from build123d import *

# Parameters (mm, degrees)
F0_R     = 50
F1_DEPTH = 10
F2_R     = 50
F2_R_2   = 45
F3_DEPTH = 200
F4_R     = 2.5
F5_DEPTH = 20


with BuildPart() as f1:
    # F0 (on Top) → F1 (new body)
    with BuildSketch(Plane.XY):
        Circle(F0_R)
    extrude(amount=F1_DEPTH)

    # F2 (on face) → F3 (join)
    with BuildSketch(Plane(origin=(0, 0, 0), x_dir=(1, 0, 0), z_dir=(0, 0, -1))):
        Circle(F2_R)
        Circle(F2_R_2, mode=Mode.SUBTRACT)
    extrude(amount=F3_DEPTH)

    # F4 (on face) → F5 (join)
    with BuildSketch(Plane.XY.offset(10)):
        Circle(F4_R)
        with Locations((-10, 0)):
            Circle(F4_R)
        with Locations((0, 10)):
            Circle(F4_R)
        with Locations((10, 0)):
            Circle(F4_R)
        with Locations((0, -10)):
            Circle(F4_R)
    extrude(amount=F5_DEPTH)


solid = f1.part
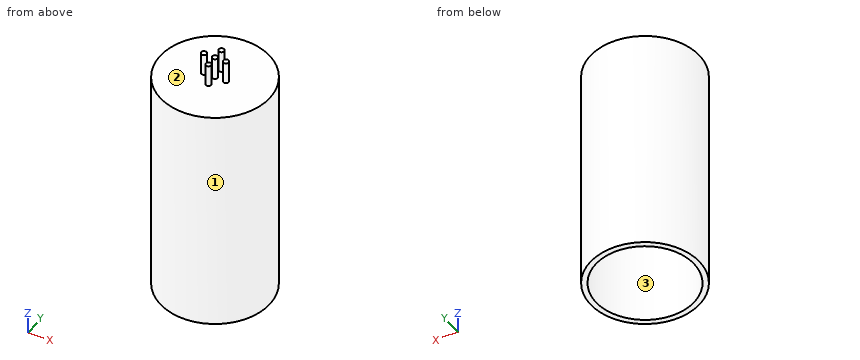
Input: part model. Units: mm. Frame: model coordinates. Face numbers are marked on the shaded views. A direction names the side the tool comes from. Coordinates: 2 decimals unless noted, no trailing zeros. Loops run counter-clockwise (first coordinate to the right, second up) from the corner with the lowest first, then second, coordinate; pieces in that order, holes last.
Q1. Material intervals for line 1 (Y direction, x = 0, z = -72); line 2 (Z direction, x = 2.5, y = -26.5), sorted ascending.
Q2. Cut plane D-D (z = 3). Output: boundary loops of the cut face in (x, y).
Q3. Cut plane B-B (y = 10). Output: boundary loops of the cut face in (x, z), then the cut area to 3 significant figures.
Q4. Set-up query: the marked faces 1, 2 and 3. Return all of +Z, -Z, +X, -X, +Y, -Y with unobstructed straight access to the full face (end or side cutting, diameter ignored); none if empty.
Q5. Cut plane A-A (x = 0). Output: boundary loops of the cut face in (y, z), then the cut area to 3 significant figures.
Q6. Cut plane C-C (z = -149.5). Output: boundary loops of the cut face in (x, y), then the cut area to 3 significant figures.
Q7. Contact query for flat-ended pins moving along their axis: pin 1 (12 mm diameter, centred on x = -29, z = -82, fed in from -Y); pin 2 (1 mm diameter, centred on x = 3, z = -148, fed in from +Y); pin 3 (4 mm diameter, centred on x = 15, y = -21, fed in from -Z). Output: stop coordinate, or through.
Working result:
1. line 1: y = -50 to -45, 45 to 50
1. line 2: z = 0 to 10
2. outline: circle Ø100 at (0, 0)
3. outline: (-48.99, -200) - (-43.87, -200) - (-43.87, 0) - (43.87, 0) - (43.87, -200) - (48.99, -200) - (48.99, 10) - (2.5, 10) - (2.5, 30) - (-2.5, 30) - (-2.5, 10) - (-48.99, 10) - close
3. area: 3,130 mm2
4. face 1: +Z, -Z
4. face 2: +Z
4. face 3: -Z
5. outline: (-50, -200) - (-45, -200) - (-45, 0) - (45, 0) - (45, -200) - (50, -200) - (50, 10) - (12.5, 10) - (12.5, 30) - (7.5, 30) - (7.5, 10) - (2.5, 10) - (2.5, 30) - (-2.5, 30) - (-2.5, 10) - (-7.5, 10) - (-7.5, 30) - (-12.5, 30) - (-12.5, 10) - (-50, 10) - close
5. area: 3,300 mm2
6. outline: circle Ø100 at (0, 0); hole circle Ø90 at (0, 0)
6. area: 1,490 mm2
7. pin 1: stops at y = -44.4
7. pin 2: stops at y = 49.94
7. pin 3: stops at z = 0
